Read the model definition and answer for the solid it produces. Units are mm, in the model's axes. Face numbers are marked on the shaded views. A direction names the side the tool comes from. Give positions to 0.01 mm unless a question says otherwise; leave off trailing zeros. Write each loop counter-clockwise with the first axis right and the second up, starting at its lowest first coordinate (ties: lowest second). Pieces come first, ordered by that corner, then holes. Notation, with made-up numbers: M -6,14.25 L 52,14.25 A26 cw 52,40.25 Z; hole C 51,-23 d10. An arc over 180 degrees is marked long. Use a Markdown table: item, result. Add a question column.
Item 1: Given P1, Ø7.5, axis at x = -39, y = -16, coming from the +Z side (3 decimals), flat-ended and moving along its own axis, determine where the tip first touches the part or whether it passes through.
Item 2: The mould has two halves that part along X. Classify the marked faces 1, 2, 3 and 4: pulls with the +X half, pulls with the -X half, needs draft (parallel to the pull), parting line crosses it, or undercut.
Item 3: A cutting plane is placed at C-C on x = -28. Determine the outline of the cut face in (y, z) (3 decimals).
Item 4: A cutting plane is placed at A-A on z = 43. Determine the outline of the cut face in (x, y), then the cut area to 3 significant figures.
Item 5: For the marked faces 5 and 6, determine the directions among +Z, -Z, +X, -X, +Y, -Y from which every point of the face is accessible in a straight line to the end or side of a thin tool.
Item 6: Consider probe 1 along X at (y, z) = (-18.5, 39); probe 2 along Z at (x, y) = (-51, -13.75) (3 decimals). Determine where each line is inside the solid, lowest interval first. Write a range as [from, to].
Item 7: A cutting plane is placed at B-B on y = -1.5. Determine the outline of the cut face in (x, z) (3 decimals), then the cut area to 3 significant figures.
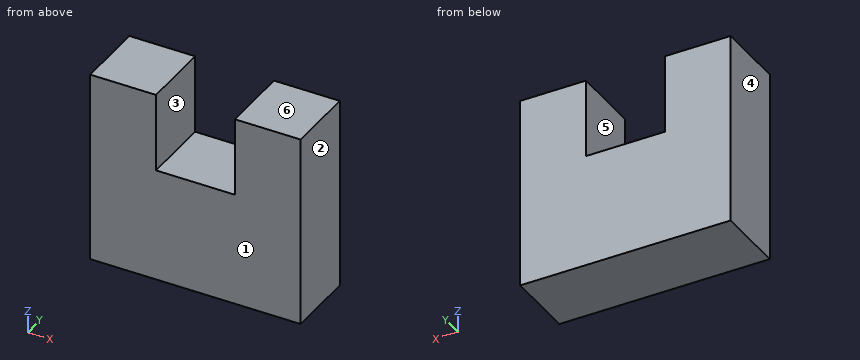
from build123d import *

# Parameters (mm, degrees)
F1_DEPTH = 25.4


with BuildPart() as f1:
    # F0 (on Front) → F1 (new body)
    with BuildSketch(Plane.XZ):
        Polygon((-23.8252, 0), (0, 0), (0, 50.8), (-23.8252, 50.8), (-23.8252, 22.225), (-52.3748, 22.225), (-52.3748, 50.8), (-76.2, 50.8), (-76.2, 0), (-52.3748, 0), align=None)
        Polygon((0, -19.05), (0, 0), (-23.8252, 0), (-52.3748, 0), (-76.2, 0), (-76.2, -19.05), align=None)
    extrude(amount=F1_DEPTH)


solid = f1.part
Filled in:
| question | item | result |
|---|---|---|
| 1 | P1 | z = 22.225 |
| 2 | face 1 | needs draft |
| 2 | face 2 | pulls with the +X half |
| 2 | face 3 | undercut |
| 2 | face 4 | pulls with the -X half |
| 3 | outline | M -25.4,-19.05 L 0,-19.05 L 0,22.225 L -25.4,22.225 Z |
| 4 | outline | M -76.2,-25.4 L -52.37,-25.4 L -52.37,0 L -76.2,0 Z; M -23.83,-25.4 L 0,-25.4 L 0,0 L -23.83,0 Z |
| 4 | area | 1,210 mm² |
| 5 | face 5 | +Z, +Y, -Y |
| 5 | face 6 | +Z, +X, -X, +Y, -Y |
| 6 | probe 1 | [-76.2, -52.37], [-23.83, 0] |
| 6 | probe 2 | [-19.05, 22.225] |
| 7 | outline | M -76.2,-19.05 L 0,-19.05 L 0,50.8 L -23.825,50.8 L -23.825,22.225 L -52.375,22.225 L -52.375,50.8 L -76.2,50.8 Z |
| 7 | area | 4,510 mm² |
